Could you check a few things on this model? Use its own coordinates, in mm. Coordinates: 2 decimals unless noted, no trailing zeros. Order: outer loops, then holes, each group sorted by start corner. A loop starts at its lowest first (then second) coordinate and runs counter-clockwise, first axis right, second up. Notation, with made-up numbers: M 38.25,14 L 77.25,14 A11 ccw 77.25,24 Z; hole C 36,40 d11. An arc over 180 degrees is marked long. Write item = value, one per line. Start each with the question number.
from build123d import *

# Parameters (mm, degrees)
ESBO_O1_W                = 40
ESBO_O1_H                = 40
RESSALTO_EXTRUS_O1_DEPTH = 1600
ESBO_O2_W                = 37
ESBO_O2_H                = 37
CORTE_EXTRUS_O1_DEPTH    = 1601


with BuildPart() as part:
    # Esboço1 → Ressalto-extrusão1 (new body)
    with BuildSketch(Plane(origin=(0, 0, 0), x_dir=(0, 0, -1), z_dir=(1, 0, 0))):
        Rectangle(ESBO_O1_W, ESBO_O1_H)
    extrude(amount=RESSALTO_EXTRUS_O1_DEPTH)

    # Esboço2 → Corte-extrusão1 (cut, through all)
    with BuildSketch(Plane.ZY):
        Rectangle(ESBO_O2_W, ESBO_O2_H)
    extrude(amount=-CORTE_EXTRUS_O1_DEPTH, mode=Mode.SUBTRACT)


solid = part.part
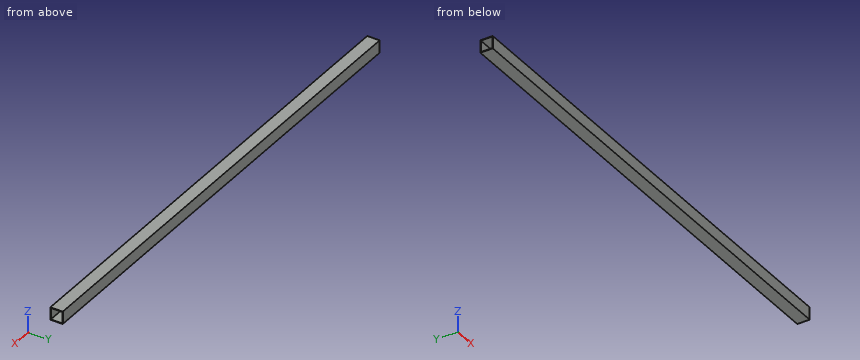
(1) Imagine slicing it at C-C on x = 1307.5. List the corners of the cut face in (y, z) for me.
(2) Please list where this line runs through material, in increasing order: probe 1 along Y at (x, z) = (137.5, 8.5). Write a range as from..to.
(3) Imagine slicing it at A-A on z = -2. List the corners of the cut face in (x, y) for me.
Response:
q1.outline = M -20,-20 L 20,-20 L 20,20 L -20,20 Z; hole M -18.5,-18.5 L 18.5,-18.5 L 18.5,18.5 L -18.5,18.5 Z
q2.probe_1 = -20..-18.5, 18.5..20
q3.outline = M 0,-20 L 1600,-20 L 1600,-18.5 L 0,-18.5 Z; M 0,18.5 L 1600,18.5 L 1600,20 L 0,20 Z
